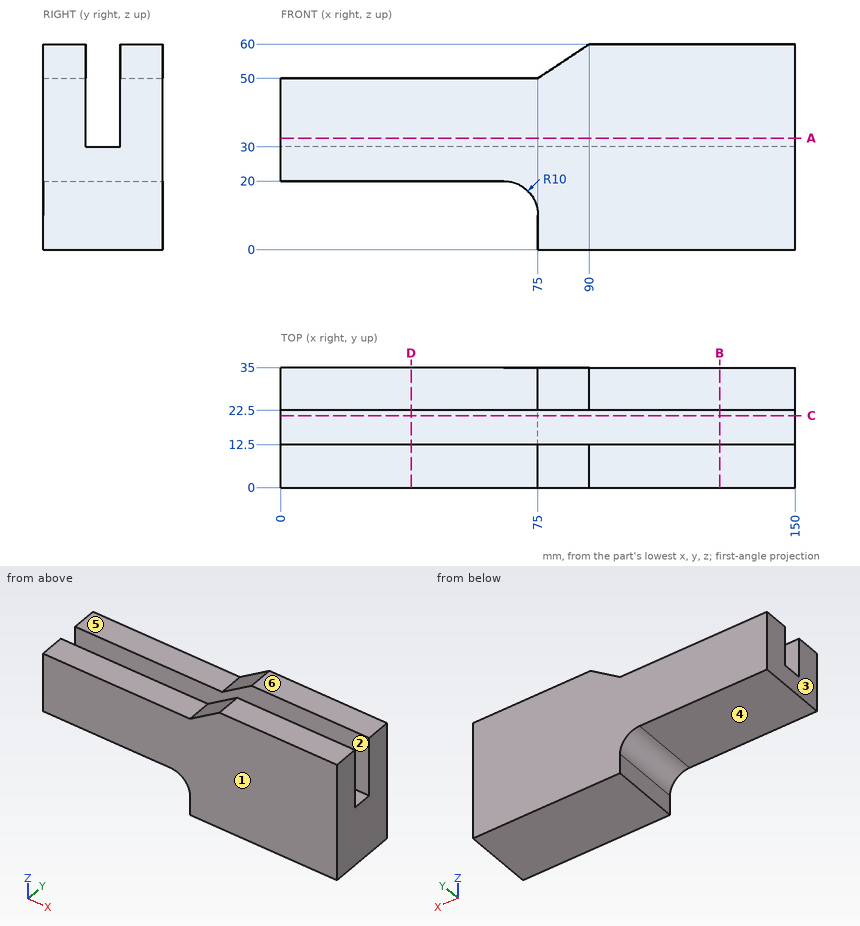
Part print with two shaded views. Sizes in mm from the minimum x, y, z corner. A direction names the side the tool comes from. Round coordinates to 2 decimals unless told otherwise and drop trailing zeros. Order: outer loops, then holes, each group sorted by start corner. A loop starts at its lowest first (then second) coordinate and runs counter-clockwise, first axis right, second up.
(1) Drill centre lines: line 1 (Y direction, x = 78, z = 31.5); line 2 (Z direction, x = 120.5, y = 13); line 3 (X direction, y = 25, z = 6.5). Where is each one in solid material? Low to high.
(2) Band-saw the part on A-A (z = 32.5). List the corners of the cut face in (x, y), then the cut area to 3 significant figures.
(3) Pull direction Y, two halves, no side cores. Call the marked faces 1, 2 and 3: released by +Y, released by -Y, zero draft, split by the parting line, or undercut.
(4) Pin check, flat tips, straight feed: pin 1 (4 mm diameter, centred on x = 50.5, y = 5.5, fed in from +Z); pin 2 (5 mm diameter, centred on x = 16, y = 9, fed in from -Z); pin 3 (5 mm diameter, centred on y = 23, z = 3.5, fed in from -X). Stop position of each tip, or through.
(5) Band-saw the part on D-D (x = 38). List the corners of the cut face in (y, z), then the cut area to 3 significant figures.
(6) Band-saw the part on C-C (y = 21). List the corners of the cut face in (x, z).
(7) Band-saw the part on B-B (x = 128). List the corners of the cut face in (y, z).
(8) 3-axis set-ups, long thin cutter, end or side, ignore diameter. For the marked faces 4, 5 and 6: which of +Z, -Z, +X, -X, +Y, -Y reach the whole face in a straight line?
Verdict:
1. line 1: y = 0 to 12.5, 22.5 to 35
1. line 2: z = 0 to 30
1. line 3: x = 75 to 150
2. outline: (0, 0) - (150, 0) - (150, 12.5) - (0, 12.5) - close; (0, 22.5) - (150, 22.5) - (150, 35) - (0, 35) - close
2. area: 3,750 mm2
3. face 1: released by -Y
3. face 2: undercut
3. face 3: zero draft
4. pin 1: stops at z = 50
4. pin 2: stops at z = 20
4. pin 3: stops at x = 75
5. outline: (0, 20) - (35, 20) - (35, 50) - (22.5, 50) - (22.5, 30) - (12.5, 30) - (12.5, 50) - (0, 50) - close
5. area: 850 mm2
6. outline: (0, 20) - (65, 20) arc R10 cw to (75, 10) - (75, 0) - (150, 0) - (150, 30) - (0, 30) - close
7. outline: (0, 0) - (35, 0) - (35, 60) - (22.5, 60) - (22.5, 30) - (12.5, 30) - (12.5, 60) - (0, 60) - close
8. face 4: -Z, -X, +Y, -Y
8. face 5: +Z, -X, +Y, -Y
8. face 6: +Z, +X, -X, +Y, -Y
